Check sheet for the modelled part. Datum: model origin and axes. Units: mm. A direction names the side the tool comes from. Coordinates: 2 decimals unless noted, no trailing zeros. Loops run counter-clockwise (first coordinate to the right, second up) from the corner with the lowest first, then second, coordinate; pieces in that order, holes last. Notation, with made-up numbers: (-12.5, 31) -> (-8.5, 31) arc R23 ccw to (-8.5, 60) -> close; hole circle Ø8 at (0.5, 56.5). An arc over 180 degrees is marked (long way). Use one line per item in the form item = value.
from build123d import *

# Parameters (mm, degrees)
SKETCH1_W           = 10
SKETCH1_H           = 10
SKETCH1_R           = 2.605
BOSS_EXTRUDE1_DEPTH = 304.8
CIRPATTERN1_COUNT   = 4
SKETCH2_R           = 2.78
CUT_EXTRUDE1_DEPTH  = 30
SKETCH3_W           = 5.08
SKETCH3_H           = 12.7
CUT_EXTRUDE2_DEPTH  = 158.75


with BuildPart() as part:
    # Sketch1 → Boss-Extrude1 (new body)
    with BuildSketch(Plane(origin=(0, 0, 0), x_dir=(0, 0, -1), z_dir=(1, 0, 0))):
        Rectangle(SKETCH1_W, SKETCH1_H)
        Circle(SKETCH1_R, mode=Mode.SUBTRACT)
        Polygon((7.474873734, 9.921463197), (2.553410537, 5), (5, 5), (5, 3.203948776), (9.596194078, 7.800142853), align=None)
        Polygon((9.596194078, 3.24), (12.596194078, 3.24), (12.596194078, 12.596194078), (3.24, 12.596194078), (3.24, 9.921463197), (7.474873734, 9.921463197), (9.596194078, 7.800142853), align=None)
    boss_extrude1 = extrude(amount=BOSS_EXTRUDE1_DEPTH)

    # CirPattern1: Boss-Extrude1 ×4 about axis
    cirpattern1_axis = Axis((0, 0, 0), (1, 0, 0))
    for i in range(1, CIRPATTERN1_COUNT):
        add(boss_extrude1.rotate(cirpattern1_axis, i * 360 / CIRPATTERN1_COUNT))

    # Sketch2 → Cut-Extrude1 (cut)
    with BuildSketch(Plane.XY.offset(12.596194078)):
        with Locations((152.4, 0)):
            Circle(SKETCH2_R)
    extrude(amount=-CUT_EXTRUDE1_DEPTH, mode=Mode.SUBTRACT)

    # Sketch3 → Cut-Extrude2 (cut)
    with BuildSketch(Plane.ZY):
        with Locations((7.381463197, 0)):
            Rectangle(SKETCH3_W, SKETCH3_H)
    extrude(amount=-CUT_EXTRUDE2_DEPTH, mode=Mode.SUBTRACT)


solid = part.part
(1) Mould release check, pull along Z, two halves, no side actions. Record for faces 1 (the flat face through (231, 0, 5)), 2 (the cylindrical face through (228.025, -1.585, 2.067)), 3 (the flat face through (150, -12.596, -8)), 4 (the flat face through (150.266, -7.495, 5.049)): +Z half, -Z half, draft (parallel to the pull), parting line (faces both ways), or undercut.
Established:
face_1 = +Z half
face_2 = undercut
face_3 = draft
face_4 = undercut
(2) Go/stop test with flat-tipped pins: P1, Ø8, axis at y = 4.5, z = -4.5, coming from the -X side; P2, Ø3, axis at x = 138.5, y = 1, coming from the -Z side. Record where each tip stops, or that it passes through.
Established:
P1 = 0
P2 = -5
(3) Section check B-B, the plane z = 0. Record the boundary of the cut face in (x, y) (3 decimals), plus the area to 3 significant figures.
Established:
outline = (0, -5) -> (304.8, -5) -> (304.8, -2.605) -> (153.371, -2.605) arc R2.78 cw to (151.429, -2.605) -> (0, -2.605) -> close; (0, 2.605) -> (151.429, 2.605) arc R2.78 cw to (153.371, 2.605) -> (304.8, 2.605) -> (304.8, 5) -> (0, 5) -> close
area = 1,460 mm²
(4) Tool access check on faces 5 (the flat face through (150, -5, 0)), 6 (the flat face through (150, 12.596, 8)), 7 (the flat face through (150, 5, 0)), 8 (the flat face through (78, 0, 4.841)), 9 (the flat face through (150, 2, -5)). Record the directions out of +Z, -Z, +X, -X, +Y, -Y that give a thin tool (end or side, any length) a straight path to the whole face; none if there is none.
Established:
face_5 = +X, -X, -Y
face_6 = +Z, -Z, +X, -X, +Y
face_7 = +X, -X, +Y
face_8 = -X
face_9 = -Z, +X, -X
(5) Section check A-A, the plane y = 0. Record the boundary of the cut face in (x, z) (3 decimals), plus the area to 3 significant figures.
Established:
outline = (0, -5) -> (149.62, -5) -> (149.62, -2.605) -> (0, -2.605) -> close; (0, 2.605) -> (149.62, 2.605) -> (149.62, 4.841) -> (0, 4.841) -> close; (155.18, -5) -> (304.8, -5) -> (304.8, -2.605) -> (155.18, -2.605) -> close; (155.18, 2.605) -> (304.8, 2.605) -> (304.8, 5) -> (158.75, 5) -> (158.75, 4.841) -> (155.18, 4.841) -> close
area = 1,410 mm²
(6) Scan lines: line 1 along Y through (x, z) = (186, 0.5); line 2 along Z through (x, y) = (109, 0) (3 decimals); line 3 along Y through (x, z) = (170.5, 11). Record each from-to range of solid material in increasing order.
Established:
line_1 = -5 to -2.56, 2.56 to 5
line_2 = -5 to -2.605, 2.605 to 4.841
line_3 = -12.6 to -3.24, 3.24 to 12.6
